```python
from build123d import *


with BuildPart() as part:
    # Sketch1 → Revolve1 (revolve)
    with BuildSketch(Plane.XY, mode=Mode.PRIVATE) as revolve1_sk:
        with BuildLine():
            Line((-3.175, 2.38125), (3.175, 2.38125))
            Line((3.175, 2.38125), (3.175, 3.96875))
            ThreePointArc((3.175, 3.96875), (2.710032015, 5.091282015), (1.5875, 5.55625))
            Line((1.5875, 5.55625), (1.5875, 3.96875))
            Line((1.5875, 3.96875), (-1.5875, 3.96875))
            Line((-1.5875, 3.96875), (-1.5875, 5.55625))
            ThreePointArc((-1.5875, 5.55625), (-2.710032015, 5.091282015), (-3.175, 3.96875))
            Line((-3.175, 3.96875), (-3.175, 2.38125))
        make_face()
    revolve(revolve1_sk.sketch.rotate(Axis((-4.911678735, 0, 0), (1, 0, 0)), 90), axis=Axis((-4.911678735, 0, 0), (1, 0, 0)))


solid = part.part
```
CAD build for the part. Positions are in the model's coordinates, mm. A direction names the side the tool comes from. Give positions to 0.01 mm unless a question says otherwise; leave off trailing zeros. Write each loop counter-clockwise with the first axis right and the second up, starting at its lowest first coordinate (ties: lowest second). Pieces come first, ordered by that corner, then holes. Notation, with made-up numbers: (21, 19.25) -> (64, 19.25) arc R20 cw to (64, 42.25) -> close; hole circle Ø3 at (-27, 66.5). An arc over 180 degrees is marked (long way). Write each question's results on one line, items separated by ' | '.
1. Two-plate mould, pull along X, no slides. Class faces 3 (the flat face through (3.175, 2, -2)), 4 (the flat face through (1.587, -1, -4)), 5 (the cylindrical face through (0.044, 2.325, -0.516)): pulls with the +X half, pulls with the -X half, needs draft (parallel to the pull), parting line crosses it, or undercut.
Geometry check:
face 3: pulls with the +X half | face 4: undercut | face 5: needs draft
2. Which spindle directions (+Z, -Z, +X, -X, +Y, -Y) get a long thin tool onto all of the face, cutting with end or side? Do faces 1 (the cylindrical face through (-0.022, 3.874, -0.86)), 2 (the flat face through (-3.175, 2, 2)). Say none if no direction does.
Geometry check:
face 1: none | face 2: +Z, -Z, -X, +Y, -Y
3. Cut at A-A, the plane z = 0. Write the cut outline in (x, y) (1 decimal).
Geometry check:
outline: (-3.2, -4) arc R1.6 ccw to (-1.6, -5.6) -> (-1.6, -4) -> (1.6, -4) -> (1.6, -5.6) arc R1.6 ccw to (3.2, -4) -> (3.2, -2.4) -> (-3.2, -2.4) -> close; (-3.2, 2.4) -> (3.2, 2.4) -> (3.2, 4) arc R1.6 ccw to (1.6, 5.6) -> (1.6, 4) -> (-1.6, 4) -> (-1.6, 5.6) arc R1.6 ccw to (-3.2, 4) -> close
4. Cut at C-C, the plane x = 0. Write the cut outline in (y, z), then the cut area to 3 significant figures.
Geometry check:
outline: circle Ø7.94 at (0, 0); hole circle Ø4.76 at (0, 0) | area: 31.7 mm²
5. Wall check: probe 1 along Y at (x, z) = (-1.25, 0); probe 2 along X at (y, z) = (0.75, -4); probe 3 along X at (y, z) = (1, 5). Give the ranges that are in metal, low to high. Write a range as [from, to].
Geometry check:
probe 1: [-3.97, -2.38], [2.38, 3.97] | probe 2: [-3.17, -1.59], [1.59, 3.17] | probe 3: [-2.7, -1.59], [1.59, 2.7]
6. Cut at D-D, the plane x = 1.75. Write the cut outline in (y, z).
Geometry check:
outline: circle Ø11.1 at (0, 0); hole circle Ø4.76 at (0, 0)
